Here's how the part is built. I have some questions about the finished solid (model axes, mm). Give positions to 0.01 mm unless a question says otherwise; leave off trailing zeros. Loops run counter-clockwise (first coordinate to the right, second up) from the corner with the lowest first, then second, coordinate; pieces in that order, holes last. Notation, with made-up numbers: (26, -8.75) - (74, -8.75) arc R18 cw to (74, 9.25) - close; hole circle Ø2 at (58.5, 64). An arc over 180 degrees is marked (long way). Return JSON: item names as keys, results as strings. Group by question number.
(1) If we section it at D-D (x = 48): Please give me the cut outline in (y, z).
(2) If we section it at B-B (z = 14): Please give me the cut outline in (x, y).
(3) For P1, Ø0.9, axis at x = 63, z = 56.5, coming from the +Y side; P2, Ø5, axis at x = 55, z = 16.5, coming from the +Y side; P3, Ø8, axis at y = 10, z = 50, coming from the -X side, each with a flat end and sliding along its axis, tell me the tip position at first contact or that it passes through.
(4) I need wall thicknesses on probe 1 along Y at (x, z) = (47, 13.5); probe 2 along Y at (x, z) = (7.5, 63); probe 3 along Y at (x, z) = (8.5, 21). Which ranges of each line are inside material? Lowest first, please. Write a range as [from, to].
(5) If we section it at A-A (x = 20): Please give me the cut outline in (y, z).
(6) If we section it at C-C (y = 28.5): Please give me the cut outline in (x, z), then the cut area to 3 significant figures.
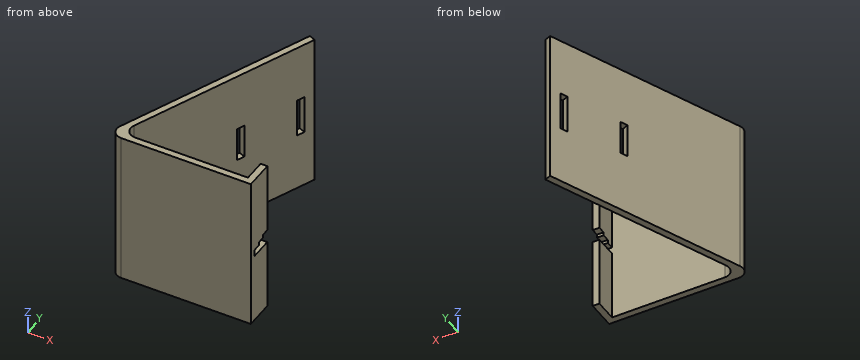
```python
from build123d import *

# Parameters (mm, degrees)
PAD_DEPTH       = 70
SKETCH001_W     = 3.5
SKETCH001_H     = 17.5
SKETCH001_H_2   = 15.5
POCKET_DEPTH    = 36.998994
POCKET001_DEPTH = 5


with BuildPart() as part:
    # Sketch → Pad (new body)
    with BuildSketch(Plane.XY):
        with BuildLine():
            Line((6.674721, 0), (65, 0))
            Line((65, 0), (65, 3))
            Line((65, 3), (65, 13))
            Line((65, 13), (62, 13))
            Line((62, 13), (62, 3))
            Line((62, 3), (11.215347, 3))
            ThreePointArc((7.158765, 9.139809), (7.535908, 4.978987), (11.215347, 3))
            Line((7.158765, 9.139809), (41.984267, 90.809258))
            Line((41.984267, 90.809258), (39.224687, 91.985998))
            Line((2.618138, 6.139809), (39.224687, 91.985998))
            ThreePointArc((2.618138, 6.139809), (2.995281, 1.978987), (6.674721, 0))
        make_face()
    extrude(amount=PAD_DEPTH)

    # Sketch001 (on Face9 of Pad) → Pocket (cut, through all)
    with BuildSketch(Plane(origin=(2.75958, -1.176741, 0), x_dir=(0.392247, 0.91986, 0), z_dir=(0.91986, -0.392247, 0))):
        with Locations((93.25, 35)):
            Rectangle(SKETCH001_W, SKETCH001_H)
        with Locations((63.75, 36)):
            Rectangle(SKETCH001_W, SKETCH001_H_2)
    extrude(amount=-POCKET_DEPTH, mode=Mode.SUBTRACT)

    # Sketch002 (on Face16 of Pocket) → Pocket001 (cut)
    with BuildSketch(Plane.YZ.offset(65)):
        Polygon((3, 35), (3, 32), (13, 32), (13, 38), (9.666667, 38), (9.666667, 36.5), (6.333333, 36.5), (6.333333, 35), align=None)
    extrude(amount=-POCKET001_DEPTH, mode=Mode.SUBTRACT)


solid = part.part
```
Values:
{
 "1": {"outline": "(0, 0) - (3, 0) - (3, 70) - (0, 70) - close"},
 "2": {"outline": "(2.62, 6.14) arc R4.41 ccw to (6.67, 0) - (65, 0) - (65, 13) - (62, 13) - (62, 3) - (11.22, 3) arc R4.41 cw to (7.16, 9.14) - (41.98, 90.81) - (39.22, 91.99) - close"},
 "3": {"P1": "y = 13", "P2": "y = 3", "P3": "x = 2.56"},
 "4": {"probe 1": "[0, 3]", "probe 2": "[0, 5.03], [9.94, 17.59]", "probe 3": "[0, 3.94], [12.29, 19.93]"},
 "5": {"outline": "(0, 0) - (3, 0) - (3, 70) - (0, 70) - close; (39.25, 0) - (46.9, 0) - (46.9, 70) - (39.25, 70) - close"},
 "6": {"outline": "(12.15, 0) - (15.41, 0) - (15.41, 70) - (12.15, 70) - close", "area": "228 mm2"}
}
